CAD build for the part. Positions are in the model's coordinates, mm. A direction names the side the tool comes from. Give positions to 0.01 mm unless a question says otherwise; leave off trailing zeros. Loops run counter-clockwise (first coordinate to the right, second up) from the corner with the lowest first, then second, coordinate; pieces in that order, holes last. Notation, with made-up numbers: (-4.75, 60.5) -> (2.25, 60.5) arc R14 cw to (2.25, 79.5) -> close; hole circle Ø9 at (63.25, 10.25). An arc over 180 degrees is marked (long way). Use one line per item in the form item = value.
```python
from build123d import *

# Parameters (mm, degrees)
SALIENTE_EXTRUIR1_DEPTH = 18.68
SALIENTE_EXTRUIR2_DEPTH = 18.68
CROQUIS3_W              = 12.25
CROQUIS3_H              = 2.83
CORTAR_EXTRUIR1_DEPTH   = 59.051339796
CROQUIS4_R              = 1.175
CORTAR_EXTRUIR2_DEPTH   = 63.813572819
CORTAR_EXTRUIR3_DEPTH   = 14.68
CROQUIS6_R              = 1
CORTAR_EXTRUIR4_DEPTH   = 5


with BuildPart() as part:
    # Croquis1 → Saliente-Extruir1 (new body)
    with BuildSketch(Plane(origin=(0, 0, 0), x_dir=(1, 0, 0), z_dir=(0, 1, 0))):
        with BuildLine():
            Line((1.5, 0), (50.6, 0))
            ThreePointArc((50.6, 0), (51.660660172, 0.439339828), (52.1, 1.5))
            Line((52.1, 1.5), (52.1, 25.5))
            ThreePointArc((52.1, 25.5), (51.660660172, 26.560660172), (50.6, 27))
            Line((50.6, 27), (1.5, 27))
            ThreePointArc((1.5, 27), (0.439339828, 26.560660172), (0, 25.5))
            Line((0, 25.5), (0, 1.5))
            ThreePointArc((0, 1.5), (0.439339828, 0.439339828), (1.5, 0))
        make_face()
        with BuildLine():
            Line((7.175, 24), (44.925, 24))
            ThreePointArc((44.925, 24), (45.985660172, 23.560660172), (46.425, 22.5))
            Line((46.425, 22.5), (46.425, 4.5))
            ThreePointArc((46.425, 4.5), (45.985660172, 3.439339828), (44.925, 3))
            Line((44.925, 3), (7.175, 3))
            ThreePointArc((7.175, 3), (6.114339828, 3.439339828), (5.675, 4.5))
            Line((5.675, 4.5), (5.675, 22.5))
            ThreePointArc((5.675, 22.5), (6.114339828, 23.560660172), (7.175, 24))
        make_face(mode=Mode.SUBTRACT)
    extrude(amount=SALIENTE_EXTRUIR1_DEPTH)

    # Croquis2 → Saliente-Extruir2 (add)
    with BuildSketch(Plane(origin=(0, 18.68, 0), x_dir=(1, 0, 0), z_dir=(0, 1, 0))):
        with BuildLine():
            Line((0, 22.27), (0, 4.73))
            ThreePointArc((0, 4.73), (-1.056857895, 5.653020288), (-1.45, 7))
            Line((-1.45, 7), (-1.45, 20))
            ThreePointArc((-1.45, 20), (-1.056857895, 21.346979712), (0, 22.27))
        make_face()
        with BuildLine():
            Line((53.55, 20), (53.55, 7))
            ThreePointArc((53.55, 7), (53.156857895, 5.653020288), (52.1, 4.73))
            Line((52.1, 4.73), (52.1, 22.27))
            ThreePointArc((52.1, 22.27), (53.156857895, 21.346979712), (53.55, 20))
        make_face()
    extrude(amount=-SALIENTE_EXTRUIR2_DEPTH)

    # Croquis3 → Cortar-Extruir1 (cut, through all)
    with BuildSketch(Plane(origin=(5.675, 0, 0), x_dir=(0, 0, -1), z_dir=(1, 0, 0))):
        with Locations((13.5, 1.415)):
            Rectangle(CROQUIS3_W, CROQUIS3_H)
    extrude(amount=-CORTAR_EXTRUIR1_DEPTH, mode=Mode.SUBTRACT)

    # Croquis4 → Cortar-Extruir2 (cut, through all)
    with BuildSketch(Plane.XZ):
        with Locations(Location((49.26, -23.3125, 0), (0, 0, 270))):
            Circle(CROQUIS4_R)
        with Locations(Location((2.8375, -23.3125, 0), (0, 0, 270))):
            Circle(CROQUIS4_R)
        with Locations(Location((49.26, -3.69, 0), (0, 0, 270))):
            Circle(CROQUIS4_R)
        with Locations(Location((2.84, -3.69, 0), (0, 0, 270))):
            Circle(CROQUIS4_R)
    extrude(amount=-CORTAR_EXTRUIR2_DEPTH, mode=Mode.SUBTRACT)

    # Croquis5 → Cortar-Extruir3 (cut)
    with BuildSketch(Plane(origin=(0, 18.68, 0), x_dir=(1, 0, 0), z_dir=(0, 1, 0))):
        Polygon((2.8375, 25.6425), (0.819660809, 24.4775), (0.819660809, 22.1475), (2.8375, 20.9825), (4.855339191, 22.1475), (4.855339191, 24.4775), align=None)
        Polygon((47.244660809, 24.4775), (49.2625, 25.6425), (51.280339191, 24.4775), (51.280339191, 22.1475), (49.2625, 20.9825), (47.244660809, 22.1475), align=None)
        Polygon((49.2625, 1.3575), (51.280339191, 2.5225), (51.280339191, 4.8525), (49.2625, 6.0175), (47.244660809, 4.8525), (47.244660809, 2.5225), align=None)
        Polygon((4.855339191, 2.5225), (2.8375, 1.3575), (0.819660809, 2.5225), (0.819660809, 4.8525), (2.8375, 6.0175), (4.855339191, 4.8525), align=None)
    extrude(amount=-CORTAR_EXTRUIR3_DEPTH, mode=Mode.SUBTRACT)

    # Croquis6 → Cortar-Extruir4 (cut)
    with BuildSketch(Plane(origin=(0, 18.68, 0), x_dir=(1, 0, 0), z_dir=(0, 1, 0))):
        with Locations(Location((0.55, 18.45, 0), (0, 0, 270))):
            Circle(CROQUIS6_R)
        with Locations(Location((0.55, 8.55, 0), (0, 0, 270))):
            Circle(CROQUIS6_R)
        with Locations(Location((51.55, 8.55, 0), (0, 0, 90))):
            Circle(CROQUIS6_R)
        with Locations(Location((51.55, 18.45, 0), (0, 0, 90))):
            Circle(CROQUIS6_R)
    extrude(amount=-CORTAR_EXTRUIR4_DEPTH, mode=Mode.SUBTRACT)


solid = part.part
```
1. Cut at C-C, the plane z = -3.69. Write the cut outline in (x, y) (1 decimal), then the cut area to 3 significant figures.
Result sheet:
outline = (0, 0) -> (1.7, 0) -> (1.7, 4) -> (0.8, 4) -> (0.8, 18.7) -> (0, 18.7) -> close; (4, 0) -> (5.9, 0) -> (5.9, 18.7) -> (4.9, 18.7) -> (4.9, 4) -> (4, 4) -> close; (46.2, 0) -> (48.1, 0) -> (48.1, 4) -> (47.2, 4) -> (47.2, 18.7) -> (46.2, 18.7) -> close; (50.4, 0) -> (52.1, 0) -> (52.1, 18.7) -> (51.3, 18.7) -> (51.3, 4) -> (50.4, 4) -> close
area = 83.6 mm^2
2. Drop flat-ended pins along their axis: P1, Ø0.7, axis at y = 15, z = -3, coming from the +X side; P2, Ø2.5, axis at x = 51.55, z = -8.55, coming from the +Y side; P3, Ø0.8, axis at x = 1, y = 1.5, coming from the -Z side; P4, Ø1.2, axis at y = 11.5, z = -24, coming from the -X side. Give the stop position or say it passes through.
Result sheet:
P1 = 52.1
P2 = 18.68
P3 = -27
P4 = 0
3. Drill centre lines: line 1 (Z direction, x = 31, y = 7); line 2 (X direction, y = 15.1, z = -8.55) (3 decimals); line 3 (X direction, y = 4.75, z = -4.25). Where is each one in solid material? Low to high.
Result sheet:
line_1 = -27 to -24, -3 to 0
line_2 = -1.45 to -0.45, 1.55 to 5.675, 46.425 to 50.55, 52.55 to 53.55
line_3 = 0 to 0.82, 4.86 to 5.7, 46.4 to 47.24, 51.28 to 52.1
4. Cut at B-B, the plane z = -8.55. Write the cut outline in (x, y) (3 decimals), then the cut area to 3 significant figures.
Result sheet:
outline = (-1.45, 2.83) -> (5.675, 2.83) -> (5.675, 18.68) -> (1.55, 18.68) -> (1.55, 13.68) -> (-0.45, 13.68) -> (-0.45, 18.68) -> (-1.45, 18.68) -> close; (46.425, 0) -> (53.55, 0) -> (53.55, 18.68) -> (52.55, 18.68) -> (52.55, 13.68) -> (50.55, 13.68) -> (50.55, 18.68) -> (46.425, 18.68) -> close
area = 226 mm^2
5. Cut at D-D, the plane y = 8.25. State how many separate pieces and enclosed holes the cut face has, then the cut area to 3 significant figures.
Result sheet:
separate_pieces = 1
enclosed_holes = 5
area = 542 mm^2
6. Mould opens along X. For faces 1 (the cylindrical face through (51.65, 9.21, -0.43)), 2 (the flat face through (2, 1, -19.625)), 3 (the flat face through (50.257, 11.443, -25.068)) say: pulls with the +X half, pulls with the -X half, needs draft (parallel to the pull), parting line crosses it, or undercut.
Result sheet:
face_1 = pulls with the +X half
face_2 = needs draft
face_3 = undercut
7. Tool access for faces 4 (the flat face through (50.286, 11.443, -5.427)), 5 (the flat face through (2, 1, -7.375)), 6 (the flat face through (0, 9, -24)), 7 (the flat face through (46.425, 9, -14)): list every direction of +Z, -Z, +X, -X, +Y, -Y with a clear straight run to the whole face (end or side of a thin tool).
Result sheet:
face_4 = +Y
face_5 = -X, -Y
face_6 = -Z, -X, +Y, -Y
face_7 = +Y, -Y
8. Cut at A-A, the plane x = 11. Write the cut outline in (y, z).
Result sheet:
outline = (0, -27) -> (18.68, -27) -> (18.68, -24) -> (0, -24) -> close; (0, -3) -> (18.68, -3) -> (18.68, 0) -> (0, 0) -> close
